Study the drawing (mm; zero at the part's minimum x, y, z) and answer. A direction names the side the tool comes from. Round coordinates to 2 decimals unless told otherwise and drop trailing zeros. Loops run counter-clockwise (first coordinate to the right, second up) from the corner with the lowest first, then second, coordinate; pieces in that order, holes last. Notation, with made-up numbers: (17.25, 15) - (48.25, 15) arc R12 ccw to (48.25, 19) - close; hole circle Ø8 at (-39, -5). An arc over 180 degrees is marked (long way). One line per item, written item: value.
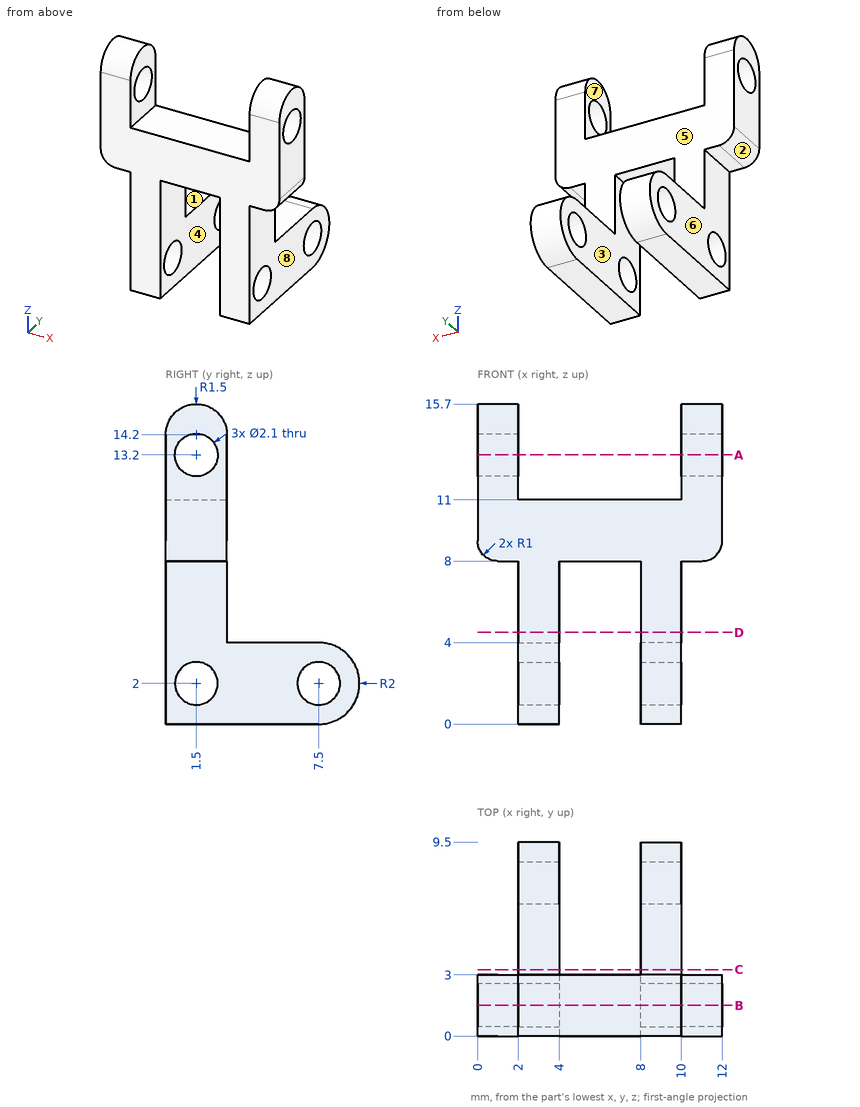
1) For a pull along X with two mould halves and no side action, classify the marked faces 1, 2 and 3 as released by +X, released by -X, zero draft, split by the parting line, or undercut.
Final values:
face 1: zero draft
face 2: released by -X
face 3: undercut
2) A cutting plane is placed at C-C on y = 3.25. Give the vertices of the cut face in (x, z).
Final values:
outline: (2, 0) - (4, 0) - (4, 4) - (2, 4) - close; (8, 0) - (10, 0) - (10, 4) - (8, 4) - close
3) For the marked faces 4, 5, 6, 7 and 8, determine the directions among +Z, -Z, +X, -X, +Y, -Y from which every point of the face is accessible in a straight line to the end or side of a thin tool.
Final values:
face 4: -Z, +Y, -Y
face 5: +Z, +X, -X, +Y
face 6: -Z, -X, +Y, -Y
face 7: +Z, +Y, -Y
face 8: -Z, +X, +Y, -Y
4) A cutting plane is placed at A-A on z = 13.2. Give the vertices of the cut face in (x, y).
Final values:
outline: (0, 0) - (2, 0) - (2, 0.45) - (0, 0.45) - close; (0, 2.55) - (2, 2.55) - (2, 3) - (0, 3) - close; (10, 0) - (12, 0) - (12, 0.45) - (10, 0.45) - close; (10, 2.55) - (12, 2.55) - (12, 3) - (10, 3) - close
5) A cutting plane is placed at D-D on z = 4.5. Give the vertices of the cut face in (x, y).
Final values:
outline: (2, 0) - (4, 0) - (4, 3) - (2, 3) - close; (8, 0) - (10, 0) - (10, 3) - (8, 3) - close
6) A cutting plane is placed at B-B on y = 1.5. Give the number of separate pieces and of enclosed holes in the cut face, and give its area (3 significant figures).
Final values:
separate pieces: 5
enclosed holes: 0
area: 69.6 mm2
7) Each of these flat-tipped pins is pushed along its axis until it touches: pin 1 Ø0.9 at (x, y) = (5, 1) entering from -Z; pin 2 Ø3.5 at (y, z) = (1.5, 13.2) entering from +X; pin 3 Ø1.9 at (y, z) = (7.5, 2) entering from -X; pin 4 Ø3 at (x, z) = (7, 11.5) entering from +Y. Where does it stop, or does it pass through?
Final values:
pin 1: z = 8
pin 2: x = 12
pin 3: through
pin 4: y = 3
8) Consider L1, parallel to Y at x = 1.2, z = 13.2; L2, parallel to X at y = 1.75, z = 14.75; L3, parallel to Z at x = 3.1, y = 1.5. Determine where each line is inside the solid, lowest interval first.
Final values:
L1: 0 to 0.45, 2.55 to 3
L2: 0 to 2, 10 to 12
L3: 0 to 0.95, 3.05 to 11
